For this review, use the dimensioned drawing (mm, ordinates from the lowest corner) and the shaded views. A direction names the side the tool comes from. Round coordinates to 2 decimals unless told otherwise and drop trailing zeros. Order: outer loops, then holes, each group sorted by start corner. A loop starts at its lowest first (then second) coordinate and runs counter-clockwise, first axis right, second up. Notation, with made-up numbers: M -25.5,13 L -13.5,13 A20 ccw -13.5,20 Z; hole C 5.25,17.5 d3. An arc over 180 degrees is marked long. Answer as CSV lines item,"result". Start each with the question number.
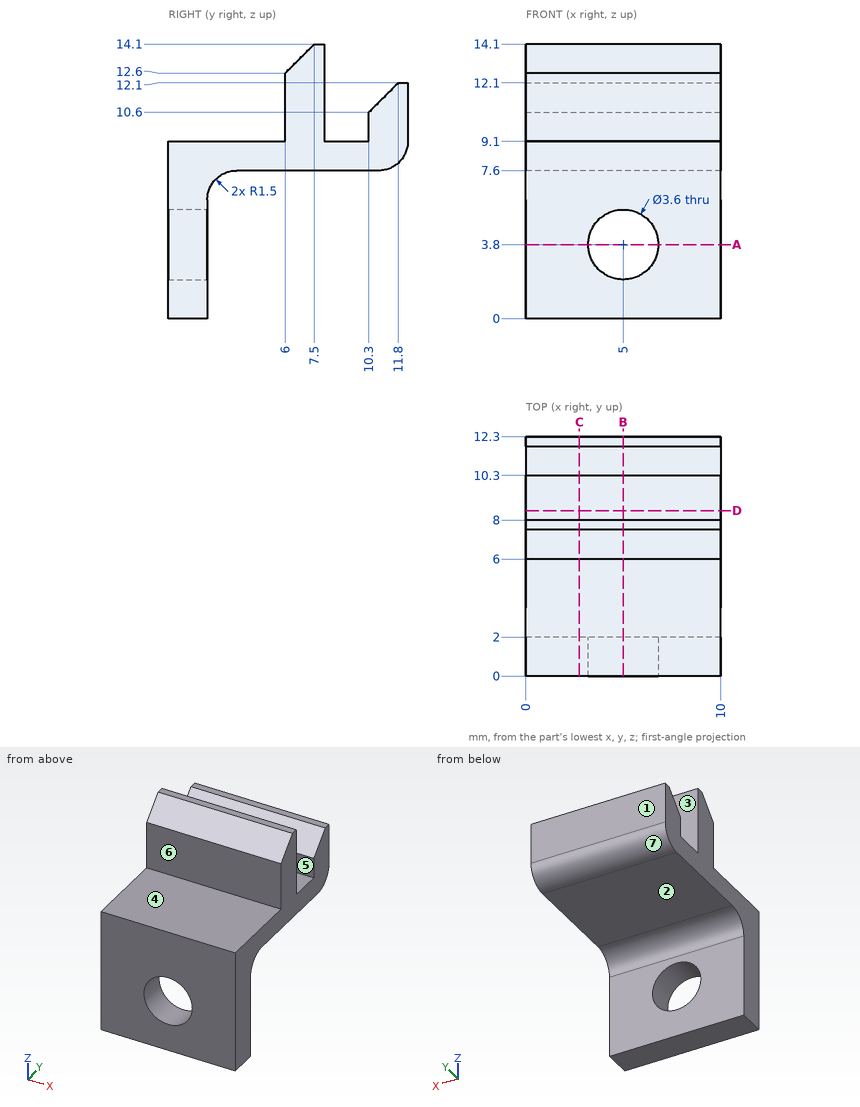
Item 1: Wall thickness on probe 1 along Z at (x, y) = (5, 0.65); probe 2 along X at (y, z) = (0.85, 3.8); probe 3 along Y at (x, z) = (1, 10): over which ranges is each line inside the solid? List them lowest first. Write a range as [from, to].
Item 2: For pin 1 (2 mm diameter, centred on x = 5.5, z = 10.5, fed in from -Y); pin 2 (6 mm diameter, centred on x = 4, y = 6.5, fed in from -Z); pin 3 (0.7 mm diameter, centred on x = 5, y = 9, fed in from +Z); pin 4 (5 mm diameter, centred on x = 6, z = 4.5, fed in from -Y), all flat-tipped, find the tip position at first contact; note any pin that passes through.
Item 3: Consider section D-D (y = 8.5). State the section outline as (x, z) points.
Item 4: Consider section C-C (x = 2.75). State the section outline as (y, z) points, and give its area (3 significant figures).
Item 5: Consider section A-A (z = 3.8). State the section outline as (x, y) points.
Item 6: The part is to be moulded in two halves that separate along Y. For the marked faces 4, 5, 6 and 7, say which applies: +Y half, -Y half, draft (parallel to the pull), parting line (faces both ways), or undercut.
Item 7: Consider section B-B (x = 5). State the section outline as (y, z) points, and give its area (3 significant figures).
Item 8: Tool access review of the marked faces 1, 2 and 3: name each direction out of +Z, -Z, +X, -X, +Y, -Y from which nothing blocks a thin tool from reaching the whole face with its end or side.
Reported:
1,probe 1,"z = [0, 2], [5.6, 9.1]"
1,probe 2,"x = [0, 3.2], [6.8, 10]"
1,probe 3,"y = [6, 8], [10.3, 12.3]"
2,pin 1,"stops at y = 6"
2,pin 2,"stops at z = 7.6"
2,pin 3,"stops at z = 9.1"
2,pin 4,"stops at y = 0"
3,outline,"M 0,7.6 L 10,7.6 L 10,9.1 L 0,9.1 Z"
4,outline,"M 0,0 L 2,0 L 2,6.1 A1.5 cw 3.5,7.6 L 10.8,7.6 A1.5 ccw 12.3,9.1 L 12.3,12.1 L 11.8,12.1 L 10.3,10.6 L 10.3,9.1 L 8,9.1 L 8,14.1 L 7.5,14.1 L 6,12.6 L 6,9.1 L 0,9.1 Z"
4,area,"47.4 mm²"
5,outline,"M 0,0 L 3.2,0 L 3.2,2 L 0,2 Z; M 6.8,0 L 10,0 L 10,2 L 6.8,2 Z"
6,face 4,"draft"
6,face 5,"undercut"
6,face 6,"-Y half"
6,face 7,"+Y half"
7,outline,"M 0,0 L 2,0 L 2,2 L 0,2 Z; M 0,5.6 L 2,5.6 L 2,6.1 A1.5 cw 3.5,7.6 L 10.8,7.6 A1.5 ccw 12.3,9.1 L 12.3,12.1 L 11.8,12.1 L 10.3,10.6 L 10.3,9.1 L 8,9.1 L 8,14.1 L 7.5,14.1 L 6,12.6 L 6,9.1 L 0,9.1 Z"
7,area,"40.2 mm²"
8,face 1,"+Z, -Z, +X, -X, +Y"
8,face 2,"-Z, +X, -X, +Y"
8,face 3,"+Z, +X, -X"
